```python
from build123d import *
from OCP.BRepFilletAPI import BRepFilletAPI_MakeChamfer

# Parameters (mm, degrees)
SKETCH1_W                      = 30
SKETCH1_H                      = 30
SKETCH1_R                      = 9.525
BOSS_EXTRUDE1_DEPTH            = 15
CHAMFER2_SIZE                  = 0.5
CHAMFER2_SIZE2                 = 0.866025404
CHAMFER3_SIZE                  = 0.5
M3X0_5_TAPPED_HOLE1_AT_2_COUNT = 2
M3X0_5_TAPPED_HOLE1_AT_2_PITCH = 20
M3X0_5_TAPPED_HOLE1_AT_3_COUNT = 2
M3X0_5_TAPPED_HOLE1_AT_3_PITCH = 10
M3X0_5_TAPPED_HOLE1_AT_4_COUNT = 2
M3X0_5_TAPPED_HOLE1_AT_4_PITCH = 10
M3X0_5_TAPPED_HOLE1_AT_5_COUNT = 2
M3X0_5_TAPPED_HOLE1_AT_5_PITCH = 10
M3X0_5_TAPPED_HOLE1_AT_6_COUNT = 2
M3X0_5_TAPPED_HOLE1_AT_6_PITCH = 22.360679775
M3X0_5_TAPPED_HOLE1_AT_7_COUNT = 2
M3X0_5_TAPPED_HOLE1_AT_7_PITCH = 22.360679775
M3X0_5_TAPPED_HOLE1_AT_8_COUNT = 2
M3X0_5_TAPPED_HOLE1_AT_8_PITCH = 14.142135624
M3X0_5_TAPPED_HOLE1_AT_9_COUNT = 2
M3X0_5_TAPPED_HOLE1_AT_9_PITCH = 14.142135624
CIRPATTERN1_COUNT              = 2


with BuildPart() as part:
    # Sketch1 → Boss-Extrude1 (new, symmetric)
    with BuildSketch(Plane.XY):
        Rectangle(SKETCH1_W, SKETCH1_H)
        Circle(SKETCH1_R, mode=Mode.SUBTRACT)
    extrude(amount=BOSS_EXTRUDE1_DEPTH, both=True)

    # Chamfer2: one chamfer whose edges measure the first distance from different faces: ONE call of the kernel's chamfer builder (chamfer() names one face for all edges)
    chamfer2_edges_1 = [part.edges().sort_by_distance(p)[0] for p in [
        (-9.525, 0, -15),
    ]]
    chamfer2_side_1 = [part.faces().sort_by_distance(p)[0] for p in [
        (0, -14.575735931, -15),
    ]]
    chamfer2_edges_2 = [part.edges().sort_by_distance(p)[0] for p in [
        (-9.525, 0, 15),
    ]]
    chamfer2_side_2 = [part.faces().sort_by_distance(p)[0] for p in [
        (-9.525, 0, 0),
    ]]
    chamfer2 = BRepFilletAPI_MakeChamfer(part.part.solid().wrapped)
    for e in chamfer2_edges_1:
        chamfer2.Add(CHAMFER2_SIZE, CHAMFER2_SIZE2, e.wrapped, chamfer2_side_1[0].wrapped)  # the first distance lies on this face
    for e in chamfer2_edges_2:
        chamfer2.Add(CHAMFER2_SIZE, CHAMFER2_SIZE2, e.wrapped, chamfer2_side_2[0].wrapped)  # the first distance lies on this face
    add(Compound.cast(chamfer2.Shape()), mode=Mode.REPLACE)

    # Chamfer3
    chamfer3_edges = [part.edges().sort_by_distance(p)[0] for p in [
        (0, 15, -15),
        (0, -15, -15),
    ]]
    chamfer(chamfer3_edges, length=CHAMFER3_SIZE)

    # Sketch8 → M3x0.5 Tapped Hole1 (revolve, cut)
    with BuildSketch(Plane(origin=(-10, 15, 0), x_dir=(0, 0, 1), z_dir=(1, 0, 0))):
        Polygon((0, 0), (0, 6.751075774), (1.25, 6), (1.25, 0), align=None)
    m3x0_5_tapped_hole1 = revolve(axis=Axis((-10, 21.35, 0), (0, -1, 0)), mode=Mode.SUBTRACT)

    # M3x0.5 Tapped Hole1 at 2: M3x0.5 Tapped Hole1 ×2
    with Locations(*[(i * M3X0_5_TAPPED_HOLE1_AT_2_PITCH, 0, 0) for i in range(1, M3X0_5_TAPPED_HOLE1_AT_2_COUNT)]):
        add(m3x0_5_tapped_hole1, mode=Mode.SUBTRACT)

    # M3x0.5 Tapped Hole1 at 3: M3x0.5 Tapped Hole1 ×2
    with Locations(*[(i * M3X0_5_TAPPED_HOLE1_AT_3_PITCH, 0, 0) for i in range(1, M3X0_5_TAPPED_HOLE1_AT_3_COUNT)]):
        add(m3x0_5_tapped_hole1, mode=Mode.SUBTRACT)

    # M3x0.5 Tapped Hole1 at 4: M3x0.5 Tapped Hole1 ×2
    with Locations(*[(0, 0, -i * M3X0_5_TAPPED_HOLE1_AT_4_PITCH) for i in range(1, M3X0_5_TAPPED_HOLE1_AT_4_COUNT)]):
        add(m3x0_5_tapped_hole1, mode=Mode.SUBTRACT)

    # M3x0.5 Tapped Hole1 at 5: M3x0.5 Tapped Hole1 ×2
    with Locations(*[(0, 0, i * M3X0_5_TAPPED_HOLE1_AT_5_PITCH) for i in range(1, M3X0_5_TAPPED_HOLE1_AT_5_COUNT)]):
        add(m3x0_5_tapped_hole1, mode=Mode.SUBTRACT)

    # M3x0.5 Tapped Hole1 at 6: M3x0.5 Tapped Hole1 ×2
    with Locations(*[Vector(0.894427190999916, 0, -0.44721359549995787) * (i * M3X0_5_TAPPED_HOLE1_AT_6_PITCH) for i in range(1, M3X0_5_TAPPED_HOLE1_AT_6_COUNT)]):
        add(m3x0_5_tapped_hole1, mode=Mode.SUBTRACT)

    # M3x0.5 Tapped Hole1 at 7: M3x0.5 Tapped Hole1 ×2
    with Locations(*[Vector(0.8944271909999159, 0, 0.447213595499958) * (i * M3X0_5_TAPPED_HOLE1_AT_7_PITCH) for i in range(1, M3X0_5_TAPPED_HOLE1_AT_7_COUNT)]):
        add(m3x0_5_tapped_hole1, mode=Mode.SUBTRACT)

    # M3x0.5 Tapped Hole1 at 8: M3x0.5 Tapped Hole1 ×2
    with Locations(*[Vector(0.7071067811865476, 0, -0.7071067811865475) * (i * M3X0_5_TAPPED_HOLE1_AT_8_PITCH) for i in range(1, M3X0_5_TAPPED_HOLE1_AT_8_COUNT)]):
        add(m3x0_5_tapped_hole1, mode=Mode.SUBTRACT)

    # M3x0.5 Tapped Hole1 at 9: M3x0.5 Tapped Hole1 ×2
    with Locations(*[Vector(0.7071067811865475, 0, 0.7071067811865476) * (i * M3X0_5_TAPPED_HOLE1_AT_9_PITCH) for i in range(1, M3X0_5_TAPPED_HOLE1_AT_9_COUNT)]):
        add(m3x0_5_tapped_hole1, mode=Mode.SUBTRACT)

    # CirPattern1: M3x0.5 Tapped Hole1 ×2 about axis
    cirpattern1_axis = Axis((0, 0, 15), (0, 0, -1))
    for i in range(1, CIRPATTERN1_COUNT):
        add(m3x0_5_tapped_hole1.rotate(cirpattern1_axis, i * 360 / CIRPATTERN1_COUNT), mode=Mode.SUBTRACT)

    # CirPattern1 copy 1 sketch → CirPattern1 copy 1 (revolve, cut)
    with BuildSketch(Plane(origin=(-10, -15, 0), x_dir=(0, 0, 1), z_dir=(-1, 0, 0))):
        Polygon((0, 0), (0, 6.751075774), (1.25, 6), (1.25, 0), align=None)
    revolve(axis=Axis((-10, -21.35, 0), (0, 1, 0)), mode=Mode.SUBTRACT)

    # CirPattern1 copy 2 sketch → CirPattern1 copy 2 (revolve, cut)
    with BuildSketch(Plane(origin=(0, -15, 0), x_dir=(0, 0, 1), z_dir=(-1, 0, 0))):
        Polygon((0, 0), (0, 6.751075774), (1.25, 6), (1.25, 0), align=None)
    revolve(axis=Axis((0, -21.35, 0), (0, 1, 0)), mode=Mode.SUBTRACT)

    # CirPattern1 copy 3 sketch → CirPattern1 copy 3 (revolve, cut)
    with BuildSketch(Plane(origin=(10, -15, -10), x_dir=(0, 0, 1), z_dir=(-1, 0, 0))):
        Polygon((0, 0), (0, 6.751075774), (1.25, 6), (1.25, 0), align=None)
    revolve(axis=Axis((10, -21.35, -10), (0, 1, 0)), mode=Mode.SUBTRACT)

    # CirPattern1 copy 4 sketch → CirPattern1 copy 4 (revolve, cut)
    with BuildSketch(Plane(origin=(10, -15, 10), x_dir=(0, 0, 1), z_dir=(-1, 0, 0))):
        Polygon((0, 0), (0, 6.751075774), (1.25, 6), (1.25, 0), align=None)
    revolve(axis=Axis((10, -21.35, 10), (0, 1, 0)), mode=Mode.SUBTRACT)

    # CirPattern1 copy 5 sketch → CirPattern1 copy 5 (revolve, cut)
    with BuildSketch(Plane(origin=(-10, -15, -10), x_dir=(0, 0, 1), z_dir=(-1, 0, 0))):
        Polygon((0, 0), (0, 6.751075774), (1.25, 6), (1.25, 0), align=None)
    revolve(axis=Axis((-10, -21.35, -10), (0, 1, 0)), mode=Mode.SUBTRACT)

    # CirPattern1 copy 6 sketch → CirPattern1 copy 6 (revolve, cut)
    with BuildSketch(Plane(origin=(-10, -15, 10), x_dir=(0, 0, 1), z_dir=(-1, 0, 0))):
        Polygon((0, 0), (0, 6.751075774), (1.25, 6), (1.25, 0), align=None)
    revolve(axis=Axis((-10, -21.35, 10), (0, 1, 0)), mode=Mode.SUBTRACT)

    # CirPattern1 copy 7 sketch → CirPattern1 copy 7 (revolve, cut)
    with BuildSketch(Plane(origin=(0, -15, -10), x_dir=(0, 0, 1), z_dir=(-1, 0, 0))):
        Polygon((0, 0), (0, 6.751075774), (1.25, 6), (1.25, 0), align=None)
    revolve(axis=Axis((0, -21.35, -10), (0, 1, 0)), mode=Mode.SUBTRACT)

    # CirPattern1 copy 8 sketch → CirPattern1 copy 8 (revolve, cut)
    with BuildSketch(Plane(origin=(0, -15, 10), x_dir=(0, 0, 1), z_dir=(-1, 0, 0))):
        Polygon((0, 0), (0, 6.751075774), (1.25, 6), (1.25, 0), align=None)
    revolve(axis=Axis((0, -21.35, 10), (0, 1, 0)), mode=Mode.SUBTRACT)


solid = part.part
```
Here's how the part is built. I have some questions about the finished solid (model axes, mm). A direction names the side the tool comes from. Round coordinates to 2 decimals unless told otherwise and drop trailing zeros. Write each loop counter-clockwise with the first axis right and the second up, starting at its lowest first coordinate (ties: lowest second). Pieces come first, ordered by that corner, then holes. Notation, with made-up numbers: M 29,87 L 63,87 A22 cw 63,115 Z; hole C 69.25,65.5 d9. An arc over 180 degrees is marked long. Answer as CSV lines item,"result". Start each with the question number.
1. Suppose I cut it at B-B on y = 0. Write out the boundary of the cut face in (x, z) (3 decimals).
2. Suppose I cut it at A-A on z = -12.75. Write out the boundary of the cut face in (x, y) (3 decimals), then the cut area to 3 significant figures.
3. Suppose I cut it at C-C on y = -11.5. Count the separate pieces of the cut face and the enclosed holes in it, then the cut area to 3 significant figures.
4. On a 3-axis mill with a long thin cutter (end or side, diameter ignored), from which of +Z, -Z, +X, -X, +Y, -Y can I reach the whole of each face in a straight line? I mean faces 4 (the cylindrical face through (11.24, -12.04, -0.16)), 5 (the cylindrical face through (-2.06, -9.3, -0.02)), 6 (the cylindrical face through (-10.845, 12.042, 9.079)). Say none if no direction works.
5. Thinking about a two-plate mould opening in X: for faces 1 (the flat face through (15, 0, 0)), 2 (the cylindrical face through (-9.95, -12.04, -11.25)), 3 (the flat face through (-10.2, 0.2, -15)), which applies, released by +X, released by -X, zero draft, split by the parting line, or undercut?
6. I need wall thicknesses on probe 1 along X at (y, z) = (13, 10); probe 2 along X at (y, z) = (-12.5, -10.5). Which ranges of each line are inside material? Lowest first, please.
7. I'm going to push flat-ended pins straight in: pin 1 Ø1.5 at (x, z) = (-10, -10) entering from +Y; pin 2 Ø3 at (x, z) = (-10, -10) entering from +Y; pin 3 Ø1.5 at (x, z) = (10, 0) entering from -Y; pin 4 Ø2 at (x, z) = (-10, 0) entering from -Y. Where does each tip first touch, or does it pass through?
Check result:
1,outline,"M -15,-15 L -10.025,-15 L -9.525,-14.134 L -9.525,14.5 L -10.391,15 L -15,15 Z; M 9.525,-14.134 L 10.025,-15 L 15,-15 L 15,15 L 10.391,15 L 9.525,14.5 Z"
2,outline,"M -15,-15 L 15,-15 L 15,15 L -15,15 Z; hole C 0,0 d19.05"
2,area,"615 mm2"
3,separate pieces,"1"
3,enclosed holes,"9"
3,area,"856 mm2"
4,face 4,"-Y"
4,face 5,"+Z, -Z"
4,face 6,"+Y"
5,face 1,"released by +X"
5,face 2,"undercut"
5,face 3,"zero draft"
6,probe 1,"x = -15 to -11.25, -8.75 to -1.25, 1.25 to 8.75, 11.25 to 15"
6,probe 2,"x = -15 to -11.15, -8.85 to -1.15, 1.15 to 8.85, 11.15 to 15"
7,pin 1,"stops at y = 8.7"
7,pin 2,"stops at y = 15"
7,pin 3,"stops at y = -8.7"
7,pin 4,"stops at y = -8.85"
